Can you work these out from the model? Positions are in its coordinate system, mm. A direction names the side the tool comes from. Round coordinates to 2 decimals unless told otherwise and drop trailing zeros. Order: outer loops, then holes, each group sorted by start corner. A loop starts at its lowest first (then second) coordinate and runs counter-clockwise, first axis right, second up. Notation, with made-up numbers: (72.5, 81.5) -> (105.5, 81.5) arc R20 ccw to (105.5, 85.5) -> close; hole circle Ø7 at (-20.75, 82.25). An arc over 180 degrees is marked (long way). Use a Markdown table: item, result. Add a question column.
Q1. If we section it at B-B on x = -2.75: List the corners of the cut face in (y, z) for me.
Q2. I'm going to push a flat-ended pin straight in: pin 1 Ø1.5 at (x, z) = (3, 1) entering from +Y. Where does the tip first touch, or does it pass through?
Q3. I need wall thicknesses on line 1 along Z through (x, y) = (-6.5, 8); line 2 along X through (y, z) = (29, 7); line 3 along Y through (x, z) = (-0.5, -8.25). Which ranges of each line are inside material? Lowest first, please. Write a range as [from, to].
Q4. If we section it at C-C on z = 9.5: List the corners of the cut face in (x, y) for me, plus the area to 3 significant figures.
Q5. If we section it at A-A on y = 41: List the corners of the cut face in (x, z) for me, plus the area to 3 significant figures.
Q6. For faces 5 (the face through (0, -7.62, 0)), 6 (the face through (1.524, 25, -7)), 7 (the face through (7, 25, 1.524)), which set-ups out of +Z, -Z, +X, -X, +Y, -Y let a thin tool reach every point of the face, with its end or its side?
Q7. We'd pull the mould along X, two halves only. Please class faces 1 (the face through (-1.588, 25, -7)), 2 (the face through (-1.587, 25, 7)), 3 (the face through (12.7, 22, -3)), 4 (the face through (-7, 50.8, -7)): +X half, -X half, draft (parallel to the pull), parting line (faces both ways), or undercut.
```python
from build123d import *

# Parameters (mm, degrees)
BOSS_EXTRUDE1_DEPTH   = 50.8
SKETCH1_W             = 11.1125
SKETCH1_H             = 11.176
BOSS_EXTRUDE1_2_DEPTH = 50.8
SKETCH1_W_2           = 11.176
BOSS_EXTRUDE1_3_DEPTH = 50.8
BOSS_EXTRUDE1_4_DEPTH = 50.8
SKETCH1_4_W           = 25.4
SKETCH1_4_H           = 25.4
BOSS_EXTRUDE2_DEPTH   = 7.62


with BuildPart() as part:
    # Sketch1 → Boss-Extrude1 (new body)
    with BuildSketch(Plane(origin=(0, 0, 0), x_dir=(1, 0, 0), z_dir=(0, 1, 0))):
        Polygon((-1.5875, 12.7), (-12.7, 12.7), (-12.7, 12.547344728), (-12.7, 1.524), (-1.5875, 1.524), align=None)
    extrude(amount=BOSS_EXTRUDE1_DEPTH)



with BuildPart() as body_2:
    # Sketch1 → Boss-Extrude1 2 (new body)
    with BuildSketch(Plane(origin=(0, 0, 0), x_dir=(1, 0, 0), z_dir=(0, 1, 0))):
        with Locations((-7.14375, -7.112)):
            Rectangle(SKETCH1_W, SKETCH1_H)
    extrude(amount=BOSS_EXTRUDE1_2_DEPTH)


with BuildPart() as body_3:
    # Sketch1 → Boss-Extrude1 3 (new body)
    with BuildSketch(Plane(origin=(0, 0, 0), x_dir=(1, 0, 0), z_dir=(0, 1, 0))):
        with Locations((7.112, 7.112)):
            Rectangle(SKETCH1_W_2, SKETCH1_H)
    extrude(amount=BOSS_EXTRUDE1_3_DEPTH)


with BuildPart() as body_4:
    # Sketch1 → Boss-Extrude1 4 (new body)
    with BuildSketch(Plane(origin=(0, 0, 0), x_dir=(1, 0, 0), z_dir=(0, 1, 0))):
        with Locations((7.112, -7.112)):
            Rectangle(SKETCH1_W_2, SKETCH1_H)
    extrude(amount=BOSS_EXTRUDE1_4_DEPTH)


with BuildPart() as part_1:
    add(part.part)

    add(body_2.part)  # Boss-Extrude2 merges body 2

    add(body_3.part)  # Boss-Extrude2 merges body 3

    add(body_4.part)  # Boss-Extrude2 merges body 4
    # Sketch1_4 → Boss-Extrude2 (add)
    with BuildSketch(Plane(origin=(0, 0, 0), x_dir=(1, 0, 0), z_dir=(0, 1, 0))):
        Rectangle(SKETCH1_4_W, SKETCH1_4_H)
    extrude(amount=-BOSS_EXTRUDE2_DEPTH)


solid = part_1.part
```
Answer below:
| question | item | result |
|---|---|---|
| 1 | outline | (-7.62, -12.7) -> (50.8, -12.7) -> (50.8, -1.52) -> (0, -1.52) -> (0, 1.52) -> (50.8, 1.52) -> (50.8, 12.7) -> (-7.62, 12.7) -> close |
| 2 | pin 1 | y = 50.8 |
| 3 | line 1 | [-12.7, -1.52], [1.52, 12.7] |
| 3 | line 2 | [-12.7, -1.59], [1.52, 12.7] |
| 3 | line 3 | [-7.62, 0] |
| 4 | outline | (-12.7, -7.62) -> (12.7, -7.62) -> (12.7, 50.8) -> (1.52, 50.8) -> (1.52, 0) -> (-1.59, 0) -> (-1.59, 50.8) -> (-12.7, 50.8) -> close |
| 4 | area | 1,330 mm² |
| 5 | outline | (-12.7, -12.7) -> (-1.59, -12.7) -> (-1.59, -1.52) -> (-12.7, -1.52) -> close; (-12.7, 1.52) -> (-1.59, 1.52) -> (-1.59, 12.7) -> (-12.7, 12.7) -> close; (1.52, -12.7) -> (12.7, -12.7) -> (12.7, -1.52) -> (1.52, -1.52) -> close; (1.52, 1.52) -> (12.7, 1.52) -> (12.7, 12.7) -> (1.52, 12.7) -> close |
| 5 | area | 498 mm² |
| 6 | face 5 | +Z, -Z, +X, -X, -Y |
| 6 | face 6 | +Z, -Z, +Y |
| 6 | face 7 | +X, -X, +Y |
| 7 | face 1 | undercut |
| 7 | face 2 | undercut |
| 7 | face 3 | +X half |
| 7 | face 4 | draft |
